from build123d import *

# Parameters (mm, degrees)
SKIZZE1_W                       = 45
SKIZZE1_H                       = 140
AUFSATZ_LINEAR_AUSTRAGEN1_DEPTH = 25
VERRUNDUNG1_R                   = 8
SKIZZE2_W                       = 50
SKIZZE2_H                       = 100
AUFSATZ_LINEAR_AUSTRAGEN2_DEPTH = 2
SKIZZE4_W                       = 10
SKIZZE4_H                       = 16.4
AUFSATZ_LINEAR_AUSTRAGEN3_DEPTH = 10.6
SKIZZE5_W                       = 44
SKIZZE5_H                       = 22
AUFSATZ_LINEAR_AUSTRAGEN4_DEPTH = 2
SKIZZE6_R                       = 4
AUFSATZ_LINEAR_AUSTRAGEN5_DEPTH = 10
VERRUNDUNG2_R                   = 0.5


with BuildPart() as part:
    # Skizze1 → Aufsatz-Linear austragen1 (new body)
    with BuildSketch(Plane(origin=(0, 0, 0), x_dir=(1, 0, 0), z_dir=(0, 1, 0))):
        Rectangle(SKIZZE1_W, SKIZZE1_H)
    extrude(amount=AUFSATZ_LINEAR_AUSTRAGEN1_DEPTH)

    # Verrundung1
    verrundung1_edges = [part.edges().sort_by_distance(p)[0] for p in [
        (-22.5, 25, 0),
        (22.5, 25, 0),
        (-22.5, 0, 0),
        (22.5, 0, 0),
    ]]
    fillet(verrundung1_edges, radius=VERRUNDUNG1_R)

    # Skizze2 → Aufsatz-Linear austragen2 (add)
    with BuildSketch(Plane(origin=(0, 25, 0), x_dir=(1, 0, 0), z_dir=(0, 1, 0))):
        Rectangle(SKIZZE2_W, SKIZZE2_H)
    extrude(amount=AUFSATZ_LINEAR_AUSTRAGEN2_DEPTH)

    # Skizze4 → Aufsatz-Linear austragen3 (add)
    with BuildSketch(Plane(origin=(0, 27, 0), x_dir=(1, 0, 0), z_dir=(0, 1, 0))):
        with Locations((-2, 41.8)):
            Rectangle(SKIZZE4_W, SKIZZE4_H)
    extrude(amount=AUFSATZ_LINEAR_AUSTRAGEN3_DEPTH)



with BuildPart() as body_2:
    # Skizze5 → Aufsatz-Linear austragen4 (new body)
    with BuildSketch(Plane(origin=(0, 27, 0), x_dir=(1, 0, 0), z_dir=(0, 1, 0))):
        Rectangle(SKIZZE5_W, SKIZZE5_H)
    extrude(amount=AUFSATZ_LINEAR_AUSTRAGEN4_DEPTH)


with BuildPart() as part_1:
    add(part.part)

    add(body_2.part)  # Aufsatz-Linear austragen5 merges body 2
    # Skizze6 → Aufsatz-Linear austragen5 (add)
    with BuildSketch(Plane(origin=(0, 29, 0), x_dir=(1, 0, 0), z_dir=(0, 1, 0))):
        with Locations(Location((17, 0, 0), (0, 0, 90))):
            Circle(SKIZZE6_R)
        with Locations(Location((-17, 0.013570227, 0), (0, 0, 90))):
            Circle(SKIZZE6_R)
    extrude(amount=AUFSATZ_LINEAR_AUSTRAGEN5_DEPTH)

    # Verrundung2
    verrundung2_edges = [part_1.edges().sort_by_distance(p)[0] for p in [
        (17, 39, 4),
        (-17, 39, 3.986429773),
    ]]
    fillet(verrundung2_edges, radius=VERRUNDUNG2_R)


solid = part_1.part
For this review, take the finished solid that the model builds, in its own axes (mm). A direction names the side the tool comes from. Give positions to 0.01 mm unless a question says otherwise; leave off trailing zeros. Loops run counter-clockwise (first coordinate to the right, second up) from the corner with the lowest first, then second, coordinate; pieces in that order, holes last.
Item 1: Tool access review of faces 1 (the flat face through (22.5, 12, 1)), 2 (the flat face through (-2, 32, -33.6)), 3 (the flat face through (0, 25, -60)), 4 (the flat face through (3, 32, -42)), 5 (the cylindrical face through (13.034, 33.684, 0.521)): name each direction out of +Z, -Z, +X, -X, +Y, -Y from which nothing blocks a thin tool from reaching the whole face with its end or side.
Item 2: Take a section at D-D, the plane x = 7. State the section outline as (y, z) points.
Item 3: Take a section at C-C, the plane x = -17. State the section outline as (y, z) points, and give its area (3 significant figures).
Item 4: Insertion check: pin 1 (10 mm diameter, centred on y = 10.5, z = -20, fed in from +X); pin 2 (8.5 mm diameter, centred on y = 32.5, z = -41.5, fed in from -X); pin 3 (3 mm diameter, centred on x = 21, z = -18.5, fed in from -Y) (3 decimals). Each pin has a flat end and moves straight along its axis. Give the tip position at first contact, or say it passes through.
Item 5: Draft analysis for pull direction Y (two halves, no side actions). For faces 6 (the flat face through (-2, 37.6, -42)), 7 (the flat face through (-7, 32, -42)), 8 (the cylindrical face through (-20.219, 22.594, -0.98)), 9 (the flat face through (20, 25, -1)), state which applies: +Y half, -Y half, draft (parallel to the pull), parting line (faces both ways), or undercut.
Item 6: Take a section at A-A, the plane y = 34. State the section outline as (x, z) points.
Item 7: For line 1 along Y through (x, z) = (3, -29.5); line 2 along X through (y, z) = (36.5, -38.5); line 3 along Z through (x, y) = (-2.5, 35), list the stretches that pass through material, from the lowest coordinate up.
Item 8: Take a section at B-B, the plane z = 58.5. State the section outline as (x, y) points.
Calculated:
1. face 1: +Z, -Z, +X, -Y
1. face 2: +X, -X, +Y
1. face 3: -Z, +X, -X, +Y
1. face 4: -Z, +X, +Y
1. face 5: +Y
2. outline: (0, -70) - (25, -70) - (25, -50) - (27, -50) - (27, -11) - (29, -11) - (29, 11) - (27, 11) - (27, 50) - (25, 50) - (25, 70) - (0, 70) - close
3. outline: (0.4, -70) - (24.6, -70) - (24.6, 70) - (0.4, 70) - close; (25, -50) - (27, -50) - (27, -11) - (29, -11) - (29, -4.01) - (38.5, -4.01) arc R0.5 ccw to (39, -3.51) - (39, 3.49) arc R0.5 ccw to (38.5, 3.99) - (29, 3.99) - (29, 11) - (27, 11) - (27, 50) - (25, 50) - close
3. area: 3,710 mm2
4. pin 1: stops at x = 22.5
4. pin 2: stops at x = -7
4. pin 3: stops at y = 1.755
5. face 6: +Y half
5. face 7: draft
5. face 8: undercut
5. face 9: undercut
6. outline: circle Ø8 at (-17, -0.01); (-7, -50) - (3, -50) - (3, -33.6) - (-7, -33.6) - close; circle Ø8 at (17, 0)
7. line 1: y = 0 to 27
7. line 2: x = -7 to 3
7. line 3: z = -50 to -33.6
8. outline: (-22.5, 8) arc R8 ccw to (-14.5, 0) - (14.5, 0) arc R8 ccw to (22.5, 8) - (22.5, 17) arc R8 ccw to (14.5, 25) - (-14.5, 25) arc R8 ccw to (-22.5, 17) - close
